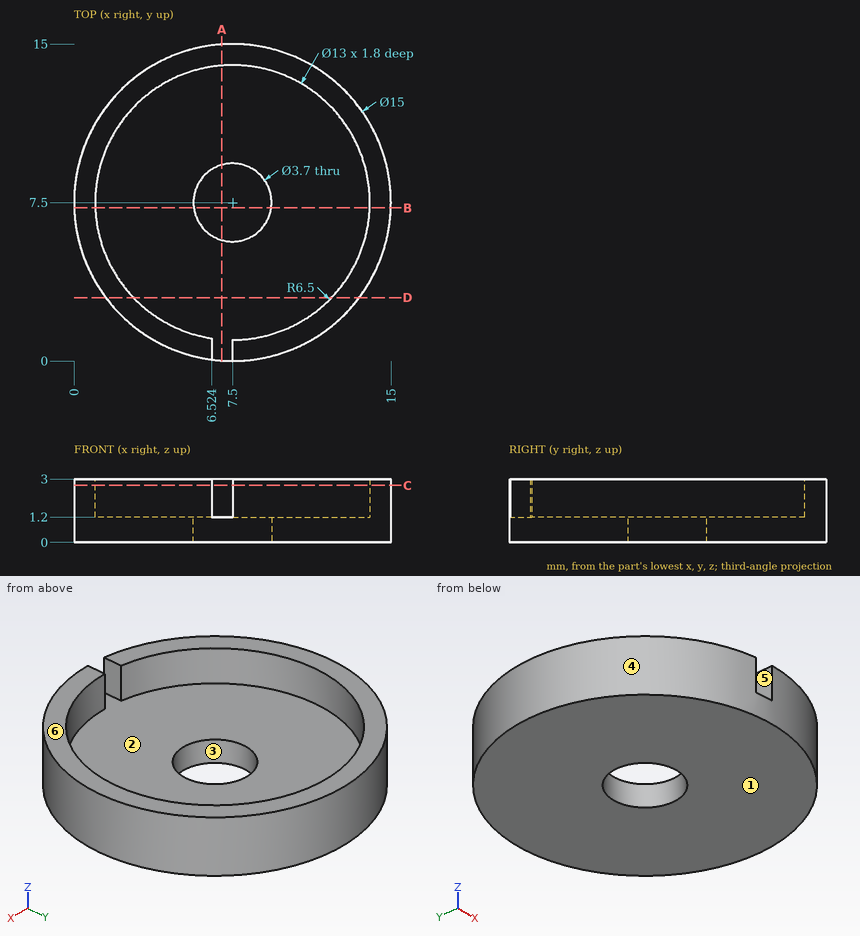
The figure shows three views and two pictorial views of one solid part (mm, origin at its lowest corner). Answer the questions. A direction names the side the tool comes from. Coordinates: 2 decimals unless noted, no trailing zeros. Write each loop counter-clockwise with the first axis right and the second up, starting at its lowest first coordinate (ties: lowest second). Pieces come first, ordered by that corner, then holes. Notation, with made-up numbers: (-5, 62.25) -> (16, 62.25) arc R21 cw to (16, 91.25) -> close; hole circle Ø3 at (77, -16.5). An arc over 180 degrees is marked (long way). Return JSON: item names as keys, results as strings.
1. Each of these flat-tipped pins is pushed along its axis until it touches: P1, Ø0.5, axis at y = 0.5, z = 2.5, coming from the -X side; P2, Ø2, axis at x = 10, y = 5, coming from the +Z side; P3, Ø1, axis at y = 10, z = 1.5, coming from the +X side. Where does it stop, or does it pass through?
Found:
{"P1": "x = 4.23", "P2": "z = 1.2", "P3": "x = 14.73"}
2. A cutting plane is placed at A-A (x = 7). Determine the outline of the cut face in (y, z), and give its area (3 significant figures).
Found:
{"outline": "(0.02, 0) -> (5.72, 0) -> (5.72, 1.2) -> (0.02, 1.2) -> close; (9.28, 0) -> (14.98, 0) -> (14.98, 3) -> (13.98, 3) -> (13.98, 1.2) -> (9.28, 1.2) -> close", "area": "15.5 mm2"}
3. A cutting plane is placed at C-C (z = 2.7). Determine the outline of the cut face in (x, y) (1 decimal).
Found:
{"outline": "(6.5, 0.1) -> (6.5, 1.1) arc R6.5 cw (long way) to (7.5, 1) -> (7.5, 0) arc R7.5 ccw (long way) to start"}
4. Find the intervals of material crossed by line 1 along X through (y, z) = (7.5, 1.7); line 2 along Z through (x, y) = (12, 7.5); line 3 along X through (y, z) = (12.75, 2.45) (1 decimal), in increasing order. Write a range as from..to.
Found:
{"line 1": "0..1, 14..15", "line 2": "0..1.2", "line 3": "2.1..3.7, 11.3..12.9"}
5. Determine the mould class of the marked faces 1, 2, 3 and 4 for opening direction Y: pulls with the +Y half, pulls with the -Y half, needs draft (parallel to the pull), parting line crosses it, or undercut.
Found:
{"face 1": "needs draft", "face 2": "undercut", "face 3": "undercut", "face 4": "parting line crosses it"}
6. A cutting plane is placed at B-B (y = 7.25). Determine the outline of the cut face in (x, z) (1 decimal).
Found:
{"outline": "(0, 0) -> (5.7, 0) -> (5.7, 1.2) -> (1, 1.2) -> (1, 3) -> (0, 3) -> close; (9.3, 0) -> (15, 0) -> (15, 3) -> (14, 3) -> (14, 1.2) -> (9.3, 1.2) -> close"}
7. A cutting plane is placed at D-D (y = 3). Determine the outline of the cut face in (x, z), and give its area (3 significant figures).
Found:
{"outline": "(1.5, 0) -> (13.5, 0) -> (13.5, 3) -> (12.19, 3) -> (12.19, 1.2) -> (2.81, 1.2) -> (2.81, 3) -> (1.5, 3) -> close", "area": "19.1 mm2"}
8. A tool of negligible diameter and unlimited length cuts with its end or side. For the marked faces 5 and 6, from which of +Z, -Z, +X, -X, +Y, -Y can it reach the whole face along a straight path? Write none if from no direction.
Found:
{"face 5": "+Z, -Y", "face 6": "+Z, +X, -X, +Y, -Y"}
